Build history of the part. All positions in model axes, mm. Face numbers are marked on the shaded views. Round coordinates to 2 decimals unless told otherwise and drop trailing zeros. Write each loop counter-clockwise with the first axis right and the second up, starting at its lowest first coordinate (ties: lowest second). Pieces come first, ordered by that corner, then holes. Notation, with made-up numbers: M 89.5,-22 L 119.5,-22 A29 ccw 119.5,16 Z; hole C 50,31.25 d3. An arc over 180 degrees is marked long. Write item = value, one per line. Start each with the question number.
Q1. Probe L1, parallel to Y at x = 6.35, z = 0.65 (3 decimals); L2, parallel to Y at x = 0, z = 1.25 (3 decimals); L3, parallel to X at y = -184.15, z = 0.75. List the from-to ranges inside material, lowest first.
Q2. Band-saw the part on A-A on x = 6.35. Write the cut outline in (y, z) (1 decimal), plus the area to 3 significant figures.
Q3. Band-saw the part on B-B on z = 0.6. State how many separate pieces and enclosed holes the cut face has, plus the area to 3 significant figures.
Q4. Pull direction Z, two halves, no side cores. Call the marked faces 1 and 2: released by +Z, released by -Z, zero draft, split by the parting line, or undercut.
Q5. Band-saw the part on D-D on x = -53.5. Write the cut outline in (y, z).
Q6. Drop a flat-ended pin along its axis: P1, Ø2.5, axis at x = 6.35, y = -184.15, coming from the +Z side. Give the stop position or say it passes through.
Q7. Band-saw the part on C-C on y = -184.15. Write the cut outline in (x, z).
Autodesk Inventor part; units mm, degrees
ref_plane "YZ Plane" through (0, 0, 0) normal (1, 0, 0) x (0, 1, 0)
ref_plane "XZ Plane" through (0, 0, 0) normal (0, 1, 0) x (-1, 0, 0)
ref_plane "XY Plane" through (0, 0, 0) normal (0, 0, 1) x (1, 0, 0)
sketch "main" plane through (0, 0, 0) normal (0, 0, 1) x (1, 0, 0)
  line L0 (38.5419, -100.052) -> (38.5419, 90.448)
  line L1 (-49.2775, -74.7747) -> (-49.2775, 55.744)
  arc A0 (-49.2775, -74.7747) -> (-40.2846, -86.9216) centre (-36.5775, -74.7747) ccw
  line L2 (13.1419, -103.227) -> (-40.2846, -86.9216)
  circle A1 centre (32.1919, -84.177) radius 2.1844
  line L3 (13.1419, -103.227) -> (35.3669, -103.227)
  arc A2 (35.3669, -103.227) -> (38.5419, -100.052) centre (35.3669, -100.052) ccw
  arc A3 (-38.4463, 76.5505) -> (-49.2775, 55.744) centre (-23.8775, 55.744) ccw
  line L4 (-18.5987, 90.448) -> (-38.4463, 76.5505)
  circle A4 centre (25.8419, 87.273) radius 2.1844
  line L5 (38.5419, 90.448) -> (-18.5987, 90.448)
  point P0 (0.4559, 3.9187)
  point P1 (-49.2775, 68.9664)
  dimension "d3" = 25.4
  dimension "d4" = 12.7
  dimension "d7" = 4.3688
sketch "Sketch1" plane through (0, 0, 0) normal (0, 0, 1) x (1, 0, 0)
  line L0 (-22.225, -9.525) -> (-22.225, -200.293)
  line L1 (12.7, -200.025) -> (12.7, -9.525)
  line L2 (-75.1194, -174.7477) -> (-75.1194, -44.2289)
  arc A0 (-75.1194, -174.7477) -> (-66.1265, -186.8946) centre (-62.4194, -174.7477) ccw
  line L3 (-12.7, -203.2) -> (-66.1265, -186.8946)
  circle A1 centre (6.35, -184.15) radius 2.1844
  line L4 (-12.7, -203.2) -> (9.525, -203.2)
  arc A2 (9.525, -203.2) -> (12.7, -200.025) centre (9.525, -200.025) ccw
  arc A3 (-64.2882, -23.4225) -> (-75.1194, -44.2289) centre (-49.7194, -44.2289) ccw
  line L5 (-44.4406, -9.525) -> (-64.2882, -23.4225)
  circle A4 centre (0, -12.7) radius 2.1844
  line L6 (12.7, -9.525) -> (-44.4406, -9.525)
  point P0 (0, 0)
extrude "Extrusion2" add sketch "Sketch1" along normal blind 1.5875
equation "\"BendRadius\" = Thickness"
equation "\"BendReliefWidth\" = Thickness"
equation "\"BendReliefDepth\" = 0.5 * Thickness"
equation "\"CornerReliefSize\" = 4 * Thickness"
equation "\"MinimumRemnant\" = 2 * Thickness"
equation "\"TransitionRadius\" = BendRadius"
equation "\"JacobiRadiusSize\" = BendRadius"
equation "\"GapSize\" = Thickness"
properties part number "wing" material "Acetal Resin, White"
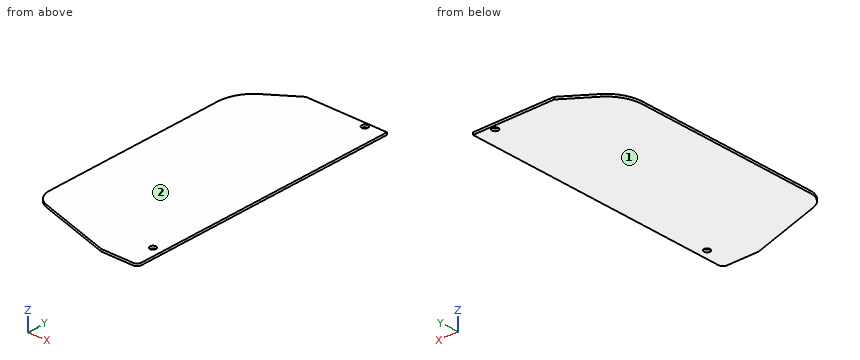
Conclusion:
q1.L1 = -203.2 to -186.334, -181.966 to -9.525
q1.L2 = -203.2 to -14.884, -10.516 to -9.525
q1.L3 = -70.96 to 4.17, 8.53 to 12.7
q2.outline = M -203.2,0 L -186.3,0 L -186.3,1.6 L -203.2,1.6 Z; M -182,0 L -9.5,0 L -9.5,1.6 L -182,1.6 Z
q2.area = 301 mm^2
q3.separate_pieces = 1
q3.enclosed_holes = 2
q3.area = 16,000 mm^2
q4.face_1 = released by -Z
q4.face_2 = released by +Z
q5.outline = M -190.75,0 L -15.87,0 L -15.87,1.59 L -190.75,1.59 Z
q6.P1 = through
q7.outline = M -70.96,0 L 4.17,0 L 4.17,1.59 L -70.96,1.59 Z; M 8.53,0 L 12.7,0 L 12.7,1.59 L 8.53,1.59 Z
